The listing builds one solid part. Answer for the finished solid, in the listing's coordinates (mm). A direction names the side the tool comes from. Coordinates: 2 decimals unless noted, no trailing zeros. Write each loop counter-clockwise with the first axis right and the second up, starting at its lowest first coordinate (ties: lowest second). Pieces come first, ordered by that corner, then holes. Notation, with made-up numbers: M 41.5,-17.75 L 74.5,-17.75 A33 ccw 74.5,16.25 Z; hole C 7,20.5 d4. An arc over 180 degrees is marked long. Put each result on its own line as item: value. Start each with the question number.
```python
from build123d import *

# Parameters (mm, degrees)
CROQUIS1_R              = 80
SALIENTE_EXTRUIR1_DEPTH = 50
SALIENTE_EXTRUIR2_DEPTH = 160
REDONDEO1_R             = 10
SALIENTE_EXTRUIR3_DEPTH = 50
CROQUIS4_R              = 60
CORTAR_EXTRUIR1_DEPTH   = 30
REDONDEO2_R             = 3


with BuildPart() as part:
    # Croquis1 → Saliente-Extruir1 (new body)
    with BuildSketch(Plane(origin=(0, 0, 0), x_dir=(1, 0, 0), z_dir=(0, 1, 0))):
        Circle(CROQUIS1_R)
        with BuildLine():
            Line((-400, -80), (0, -80))
            ThreePointArc((-1.47e-14, -80), (-80, 9.8e-15), (4.9e-15, 80))
            Line((0, 80), (-400, 80))
            Line((-400, 80), (-400, -80))
        make_face()
    extrude(amount=-SALIENTE_EXTRUIR1_DEPTH)

    # Croquis2 → Saliente-Extruir2 (add)
    with BuildSketch(Plane.XY.offset(80)):
        with BuildLine():
            Line((-400, 0), (-400, 100))
            Line((-400, 100), (-380, 100))
            ThreePointArc((-380, 100), (-321.1342666126881, 64.65443602167947), (-298.01960972814436, 0))
            Line((-298.01960972814436, 0), (-400, 0))
        make_face()
    extrude(amount=-SALIENTE_EXTRUIR2_DEPTH)

    # Redondeo1
    # the kernel refuses this fillet: 10 mm, written as the material it adds along each edge
    with BuildSketch(Plane(origin=(-298.01960972814436, -1.78e-15, 80), x_dir=(-0.04469534055522645, 0.9990006639300358, 0), z_dir=(0, 0, -1))) as redondeo1_piece_1:
        with BuildLine():
            CenterArc((9.563049951863276, 9.990006639300384), REDONDEO1_R, 182.561707770238, 84.87658445952434)
            Line((-0.4269566874370806, 9.543053233748063), (0, 0))
            ThreePointArc((0, 0), (4.5580482731555065, 0.10191268242766027), (9.11609654631102, -3e-17))
        make_face()
    extrude(amount=160)
    # the kernel refuses this fillet: 10 mm, written as the material it takes off along each edge
    with BuildSketch(Plane(origin=(0, 0, 0), x_dir=(8e-17, 0, -1), z_dir=(-1, 0, -8e-17))) as redondeo1_2_piece_1:
        with BuildLine():
            CenterArc((80 - REDONDEO1_R, REDONDEO1_R), REDONDEO1_R, 270, 90)
            Line((80 - REDONDEO1_R, -1.78e-15), (80, 0))
            Line((80, 0), (80, REDONDEO1_R))
        make_face()
    revolve(axis=Axis((0, 0, 0), (0, -1, 0)), revolution_arc=180, mode=Mode.SUBTRACT)
    with BuildSketch(Plane(origin=(-288.467010237163, 0, 80), x_dir=(0, 0, -1), z_dir=(1, 0, 0)), Plane(origin=(0, 0, -80), x_dir=(0, 0, 1), z_dir=(-1, 0, 0))) as redondeo1_2_piece_2:
        with BuildLine():
            CenterArc((REDONDEO1_R, -REDONDEO1_R), REDONDEO1_R, 90, 90)
            Line((0, -REDONDEO1_R), (0, 0))
            Line((0, 0), (REDONDEO1_R, 0))
        make_face()
    extrude(amount=288.467010237163, mode=Mode.SUBTRACT)
    with BuildSketch(Plane(origin=(-379.9999999999998, 100, 82.6745154998789), x_dir=(0.9795385270864807, -0.20125673641706543, 0), z_dir=(0, 0, -1))) as redondeo1_2_piece_3:
        with BuildLine():
            CenterArc((1.0173546356310936, 9.999862440723893), REDONDEO1_R, 258.3895408215282, 11.91098588292175)
            Line((-0.9952127285396165, 0.20447716985909684), (0, 0))
            ThreePointArc((0, 0), (0.5349030999756575, -0.00140283486632694), (1.0698061999513302, -1e-17))
        make_face()
    extrude(amount=165.34903099975782, mode=Mode.SUBTRACT)
    with BuildSketch(Plane(origin=(-400, 1.1013e-13, -80), x_dir=(-0.04779718259448206, 0.9988570615138231, 0), z_dir=(-0.9988570615138231, -0.04779718259448206, 0))) as redondeo1_2_piece_4:
        with BuildLine():
            CenterArc((101.98039027185561 - REDONDEO1_R, -REDONDEO1_R), REDONDEO1_R, 0, 90)
            Line((101.98039027185561, -REDONDEO1_R), (101.98039027185561, 0))
            Line((101.98039027185561, 0), (101.98039027185561 - REDONDEO1_R, 0))
        make_face()
    revolve(axis=Axis((-400, 1.1013e-13, -80), (0, 0, -1)), revolution_arc=87.61620511364934, mode=Mode.SUBTRACT)
    with BuildSketch(Plane(origin=(-400, 1.1013e-13, 80), x_dir=(-0.04779718259448206, 0.9988570615138231, 0), z_dir=(-0.9988570615138231, -0.04779718259448206, 0))) as redondeo1_2_piece_5:
        with BuildLine():
            CenterArc((101.98039027185561 - REDONDEO1_R, REDONDEO1_R), REDONDEO1_R, 270, 90)
            Line((101.98039027185561, REDONDEO1_R), (101.98039027185561, 0))
            Line((101.98039027185561, 0), (101.98039027185561 - REDONDEO1_R, 0))
        make_face()
    revolve(axis=Axis((-400, 1.1013e-13, 80), (0, 0, -1)), revolution_arc=87.61620511364934, mode=Mode.SUBTRACT)
    with BuildSketch(Plane(origin=(-288.467010237163, 10.000000000000012, 80), x_dir=(-0.9960046530653047, -0.0893013497784993, 0), z_dir=(-0.0893013497784993, 0.9960046530653047, 0))) as redondeo1_2_piece_6:
        with BuildLine():
            CenterArc((10.000000000000025 + REDONDEO1_R, -REDONDEO1_R), REDONDEO1_R, 90, 90)
            Line((10.000000000000025, -REDONDEO1_R), (10.000000000000025, 0))
            Line((10.000000000000025, 0), (10.000000000000025 + REDONDEO1_R, 0))
        make_face()
    revolve(axis=Axis((-288.467010237163, 10.000000000000012, 80), (0, 0, 1)), revolution_arc=84.87658445952435, mode=Mode.SUBTRACT)
    with BuildSketch(Plane(origin=(-288.467010237163, 10.000000000000012, -80), x_dir=(-0.9960046530653047, -0.0893013497784993, 0), z_dir=(-0.0893013497784993, 0.9960046530653047, 0))) as redondeo1_2_piece_7:
        with BuildLine():
            CenterArc((10.000000000000025 + REDONDEO1_R, REDONDEO1_R), REDONDEO1_R, 180, 90)
            Line((10.000000000000025, REDONDEO1_R), (10.000000000000025, 0))
            Line((10.000000000000025, 0), (10.000000000000025 + REDONDEO1_R, 0))
        make_face()
    revolve(axis=Axis((-288.467010237163, 10.000000000000012, -80), (0, 0, 1)), revolution_arc=84.87658445952435, mode=Mode.SUBTRACT)

    # Croquis3 → Saliente-Extruir3 (add)
    with BuildSketch(Plane.ZY.offset(400)):
        Polygon((44.99999999999997, -50), (24.999999999999982, -50), (25, 100), (45, 100), align=None)
        Polygon((-45, 100), (-25, 100), (-24.999999999999982, -50), (-44.99999999999997, -50), align=None)
    extrude(amount=SALIENTE_EXTRUIR3_DEPTH)

    # Croquis4 → Cortar-Extruir1 (cut)
    with BuildSketch(Plane.XZ.offset(50)):
        with Locations(Location((0, 0, 0), (0, 0, 270))):
            Circle(CROQUIS4_R)
    extrude(amount=-CORTAR_EXTRUIR1_DEPTH, mode=Mode.SUBTRACT)

    # Redondeo2
    redondeo2_edges = [part.edges().sort_by_distance(p)[0] for p in [
        (4.502e-14, -50, 60),
    ]]
    fillet(redondeo2_edges, radius=REDONDEO2_R)


solid = part.part
```
1) Straight lines are drawn through the part: probe 1 along X at (y, z) = (-38.75, 0); probe 2 along Y at (x, z) = (-258.5, 68); probe 3 along X at (y, z) = (9, -9). For each, find the intervals that lie inside material, in ascending order.
2) Determine the mould class of faces 6 (the face through (2.64, -33.69, 59.94)), 7 (the face through (-146.25, -2.85, 76.99)), 8 (the face through (-112, 0, -1)) for opening direction Z: +Z half, -Z half, draft (parallel to the pull), parting line (faces both ways), or undercut.
3) A cutting plane is placed at B-B on x = -197.5. Write down the section's boundary in (y, z), then the cut area to 3 significant figures.
4) A cutting plane is placed at A-A on z = 0. Write down the section's boundary in (x, y).
5) For faces 1 (the face through (-400, 24, 0)), 2 (the face through (-450, 26, 35)), 3 (the face through (1, -20, 1)), 4 (the face through (-400, 24, -62)), 5 (the face through (-400, 24, 63)), determine the directions among +Z, -Z, +X, -X, +Y, -Y from which every point of the face is accessible in a straight line to the end or side of a thin tool.
6) Given pin 1 Ø6 at (y, z) = (75, 39.5) entering from +X; pin 2 Ø3 at (x, z) = (-87, 49) entering from +Y; pin 3 Ø12 at (y, z) = (-13, 2.5) entering from -X, each flat-ended and moving along its own axis, determine where each tip first touches the part or whether it passes through.
Answers follow:
1. probe 1: x = -400 to -60, 60 to 80
1. probe 2: y = -50 to 0
1. probe 3: x = -400 to -298.42
2. face 6: undercut
2. face 7: +Z half
2. face 8: draft
3. outline: M -50,-80 L -10,-80 A10 ccw 0,-70 L 0,70 A10 ccw -10,80 L -50,80 Z
3. area: 7,960 mm²
4. outline: M -400,-50 L -63,-50 A3 ccw -60,-47 L -60,-20 L 60,-20 L 60,-47 A3 ccw 63,-50 L 80,-50 L 80,-10 A10 ccw 70,0 L -288.47,0 A10 cw -298.43,9.11 A101.98 ccw -378.95,99.78 A10 ccw -381.02,100 L -400,100 Z
5. face 1: -X, +Y, -Y
5. face 2: +Z, -Z, -X, +Y, -Y
5. face 3: -Y
5. face 4: -Z, -X, +Y, -Y
5. face 5: +Z, -X, +Y, -Y
6. pin 1: stops at x = -327.78
6. pin 2: stops at y = 0
6. pin 3: stops at x = -400
